Could you check a few things on this model? Use its own coordinates, in mm. A direction names the side the tool comes from. Round coordinates to 2 decimals unless told otherwise and drop trailing zeros. Loops run counter-clockwise (first coordinate to the right, second up) from the corner with the lowest first, then second, coordinate; pieces in that order, holes last. Notation, with made-up numbers: M 67,72.25 L 118,72.25 A21 ccw 118,94.25 Z; hole C -16.5,58 d10. An arc over 180 degrees is marked long. Answer in a Markdown table with one row per item.
```python
from build123d import *

# Parameters (mm, degrees)
SKETCH_1_W               = 154
SKETCH_1_H               = 37.7
EXTRUDE_1_DEPTH          = 4
CUT_EXTRUDE_1_DEPTH      = 80.374570865
CUT_EXTRUDE_1_DEPTH_BACK = 80.374570865
SKETCH_2_R               = 2
CUT_EXTRUDE_2_DEPTH      = 80.374570865
CUT_EXTRUDE_2_DEPTH_BACK = 80.374570865
FILLET_1_R               = 7
SKETCH_4_W               = 30
SKETCH_4_H               = 37.7
EXTRUDE_2_DEPTH          = 40
CUT_EXTRUDE_3_DEPTH      = 89.793707547
CUT_EXTRUDE_3_DEPTH_BACK = 89.793707547
SKETCH_5_W               = 20
SKETCH_5_H               = 11.35
CUT_EXTRUDE_4_DEPTH      = 89.793707547
CUT_EXTRUDE_4_DEPTH_BACK = 89.793707547
FILLET_2_R               = 1
FILLET_4_R               = 1


with BuildPart() as part:
    # 草图1 → 凸台-拉伸1 (new body)
    with BuildSketch(Plane(origin=(0, 0, 0), x_dir=(1, 0, 0), z_dir=(0, 1, 0))):
        Rectangle(SKETCH_1_W, SKETCH_1_H)
    extrude(amount=-EXTRUDE_1_DEPTH)

    # 草图2 → 切除-拉伸1 (cut, two sides: drawn at the far end of the back side and taken through both)
    with BuildSketch(Plane(origin=(0, 0, 0), x_dir=(1, 0, 0), z_dir=(0, 1, 0)).offset(-CUT_EXTRUDE_1_DEPTH_BACK)):
        with Locations(Location((-30, 11.85, 0), (0, 0, 270))):
            Circle(SKETCH_2_R)
        with Locations(Location((-20, -11.85, 0), (0, 0, 270))):
            Circle(SKETCH_2_R)
        with Locations(Location((-40, 11.85, 0), (0, 0, 270))):
            Circle(SKETCH_2_R)
        with Locations(Location((-50, 11.85, 0), (0, 0, 270))):
            Circle(SKETCH_2_R)
        with Locations(Location((-60, 11.85, 0), (0, 0, 270))):
            Circle(SKETCH_2_R)
        with Locations(Location((-30, -11.85, 0), (0, 0, 270))):
            Circle(SKETCH_2_R)
        with Locations(Location((-40, -11.85, 0), (0, 0, 270))):
            Circle(SKETCH_2_R)
        with Locations(Location((-50, -11.85, 0), (0, 0, 270))):
            Circle(SKETCH_2_R)
        with Locations(Location((-60, -11.85, 0), (0, 0, 270))):
            Circle(SKETCH_2_R)
        with Locations(Location((-70, -11.85, 0), (0, 0, 270))):
            Circle(SKETCH_2_R)
        with Locations(Location((20, -11.85, 0), (0, 0, 270))):
            Circle(SKETCH_2_R)
        with Locations(Location((30, -11.85, 0), (0, 0, 270))):
            Circle(SKETCH_2_R)
        with Locations(Location((40, -11.85, 0), (0, 0, 270))):
            Circle(SKETCH_2_R)
        with Locations(Location((50, -11.85, 0), (0, 0, 270))):
            Circle(SKETCH_2_R)
        with Locations(Location((60, -11.85, 0), (0, 0, 270))):
            Circle(SKETCH_2_R)
        with Locations(Location((70, -11.85, 0), (0, 0, 270))):
            Circle(SKETCH_2_R)
        with Locations(Location((30, 11.85, 0), (0, 0, 270))):
            Circle(SKETCH_2_R)
        with Locations(Location((40, 11.85, 0), (0, 0, 270))):
            Circle(SKETCH_2_R)
        with Locations(Location((50, 11.85, 0), (0, 0, 270))):
            Circle(SKETCH_2_R)
        with Locations(Location((60, 11.85, 0), (0, 0, 270))):
            Circle(SKETCH_2_R)
    extrude(amount=CUT_EXTRUDE_1_DEPTH + CUT_EXTRUDE_1_DEPTH_BACK, mode=Mode.SUBTRACT)

    # 草图3 → 切除-拉伸2 (cut, two sides: drawn at the far end of the back side and taken through both)
    with BuildSketch(Plane(origin=(0, 0, 0), x_dir=(1, 0, 0), z_dir=(0, 1, 0)).offset(-CUT_EXTRUDE_2_DEPTH_BACK)):
        Polygon((-64.644023205, 18.85), (-77, -10.433665004), (-77, 18.85), align=None)
        Polygon((64.644023205, 18.85), (77, -10.433665004), (77, 18.85), align=None)
    extrude(amount=CUT_EXTRUDE_2_DEPTH + CUT_EXTRUDE_2_DEPTH_BACK, mode=Mode.SUBTRACT)

    # 圆角1
    fillet_1_edges = [part.edges().sort_by_distance(p)[0] for p in [
        (77, -2, 18.85),
        (77, -2, 10.433665004),
        (64.644023205, -2, -18.85),
        (-77, -2, 18.85),
        (-77, -2, 10.433665004),
        (-64.644023205, -2, -18.85),
    ]]
    fillet(fillet_1_edges, radius=FILLET_1_R - 0.0001)  # a hair under: the kernel refuses the full size

    # 草图4 → 凸台-拉伸2 (add)
    with BuildSketch(Plane(origin=(0, 0, 0), x_dir=(1, 0, 0), z_dir=(0, 1, 0))):
        Rectangle(SKETCH_4_W, SKETCH_4_H)
    extrude(amount=EXTRUDE_2_DEPTH)

    # 草图5 → 切除-拉伸3 (cut, two sides: drawn at the far end of the back side and taken through both)
    with BuildSketch(Plane(origin=(0, 0, 0), x_dir=(1, 0, 0), z_dir=(0, 1, 0)).offset(-CUT_EXTRUDE_3_DEPTH_BACK)):
        with Locations((0, 8.175)):
            Rectangle(SKETCH_5_W, SKETCH_5_H)
        with Locations((0, -8.175)):
            Rectangle(SKETCH_5_W, SKETCH_5_H)
    extrude(amount=CUT_EXTRUDE_3_DEPTH + CUT_EXTRUDE_3_DEPTH_BACK, mode=Mode.SUBTRACT)

    # 草图6 → 切除-拉伸4 (cut, two sides: drawn at the far end of the back side and taken through both)
    with BuildSketch(Plane(origin=(0, 0, 0), x_dir=(1, 0, 0), z_dir=(0, 1, 0)).offset(-CUT_EXTRUDE_4_DEPTH_BACK)):
        Polygon((-34.341491259, -6.705332858), (-40, 6.705332858), (-45.658508741, -6.705332858), align=None)
        Polygon((-55.658508741, 6.705332858), (-50, -6.705332858), (-44.341491259, 6.705332858), align=None)
        Polygon((-60, 6.705332858), (-65.658508741, -6.705332858), (-54.341491259, -6.705332858), align=None)
        Polygon((-35.658508741, 6.705332858), (-30, -6.705332858), (-24.341491259, 6.705332858), align=None)
        Polygon((24.341491259, 6.705332858), (35.658508741, 6.705332858), (30, -6.705332858), align=None)
        Polygon((45.658508741, -6.705332858), (34.341491259, -6.705332858), (40, 6.705332858), align=None)
        Polygon((44.341491259, 6.705332858), (55.658508741, 6.705332858), (50, -6.705332858), align=None)
        Polygon((65.658508741, -6.705332858), (54.341491259, -6.705332858), (60, 6.705332858), align=None)
    extrude(amount=CUT_EXTRUDE_4_DEPTH + CUT_EXTRUDE_4_DEPTH_BACK, mode=Mode.SUBTRACT)

    # 圆角2
    fillet_2_edges = [part.edges().sort_by_distance(p)[0] for p in [
        (50, -2, 6.705332858),
        (44.341491259, -2, -6.705332858),
        (55.658508741, -2, -6.705332858),
        (40, -2, -6.705332858),
        (45.658508741, -2, 6.705332858),
        (34.341491259, -2, 6.705332858),
        (60, -2, -6.705332858),
        (65.658508741, -2, 6.705332858),
        (54.341491259, -2, 6.705332858),
        (-45.658508741, -2, 6.705332858),
        (-40, -2, -6.705332858),
        (-34.341491259, -2, 6.705332858),
        (-60, -2, -6.705332858),
        (-54.341491259, -2, 6.705332858),
        (-65.658508741, -2, 6.705332858),
        (-24.341491259, -2, -6.705332858),
        (-30, -2, 6.705332858),
        (-35.658508741, -2, -6.705332858),
        (-44.341491259, -2, -6.705332858),
        (-50, -2, 6.705332858),
        (-55.658508741, -2, -6.705332858),
        (30, -2, 6.705332858),
        (24.341491259, -2, -6.705332858),
        (35.658508741, -2, -6.705332858),
    ]]
    fillet(fillet_2_edges, radius=FILLET_2_R)

    # 圆角4
    fillet_4_edges = [part.edges().sort_by_distance(p)[0] for p in [
        (-15, 0, 0),
        (15, 0, 0),
    ]]
    fillet(fillet_4_edges, radius=FILLET_4_R)


solid = part.part
```
1) If we mould it in two halves opening along X, with no side actions, what happens to faces 1 (the face through (-10, 18, -8)), 2 (the face through (0, 13, 18.85)), 3 (the face through (15, 20, 0))? For each: released by +X, released by -X, zero draft, split by the parting line, or undercut.
Computed:
| item | result |
|---|---|
| face 1 | undercut |
| face 2 | zero draft |
| face 3 | released by +X |
2) I need wall thicknesses on line 1 (Z direction, x = 50, y = -1); line 2 (Z direction, x = 6, y = 11.5); line 3 (X direction, y = 34.5, z = 5). Which ranges of each line are inside material? Lowest first, please.
Computed:
| item | result |
|---|---|
| line 1 | z = -18.85 to -13.85, -9.85 to -6.71, 5.13 to 9.85, 13.85 to 18.85 |
| line 2 | z = -18.85 to -13.85, -2.5 to 2.5, 13.85 to 18.85 |
| line 3 | x = -15 to -10, 10 to 15 |
3) I want a section at C-C, the plane z = -12. State how many separate pieces and enclosed holes the cut face has, plus the area to 3 significant figures.
Computed:
| item | result |
|---|---|
| separate pieces | 10 |
| enclosed holes | 0 |
| area | 733 mm² |
4) Which directions (+Z, -Z, +X, -X, +Y, -Y) give clear straight access to the entire face, cutting with the end or side of a thin tool? Please do faces 4 (the face through (42.97, -2.03, 0.33)), 5 (the face through (-71.38, -2.03, -2.89)).
Computed:
| item | result |
|---|---|
| face 4 | +Y, -Y |
| face 5 | -Z, -X, +Y, -Y |
5) Will these pins go through, and if not, where does the flat tip stop? P1, Ø3, axis at x = -40, z = 11.85, coming from the -Y side; P2, Ø12, axis at x = -16.5, y = 15.5, coming from the -Z side; P3, Ø3.5, axis at y = 10, z = 8, coming from the -X side; P4, Ø12.5, axis at y = 9, z = 8, coming from the +X side.
Computed:
| item | result |
|---|---|
| P1 | passes through |
| P2 | stops at z = -18.85 |
| P3 | stops at x = -15 |
| P4 | stops at x = 15 |
6) I want a section at B-B, the plane y = 11. Please give me the cut outline in (x, z).
Computed:
| item | result |
|---|---|
| outline | M -15,-18.85 L 15,-18.85 L 15,18.85 L -15,18.85 Z; hole M -10,-13.85 L 10,-13.85 L 10,-2.5 L -10,-2.5 Z; hole M -10,2.5 L 10,2.5 L 10,13.85 L -10,13.85 Z |
7) I want a section at A-A, the plane x = -6. Please give me the cut outline in (y, z), plus the area to 3 significant figures.
Computed:
| item | result |
|---|---|
| outline | M -4,-18.85 L 40,-18.85 L 40,-13.85 L -4,-13.85 Z; M -4,-2.5 L 40,-2.5 L 40,2.5 L -4,2.5 Z; M -4,13.85 L 40,13.85 L 40,18.85 L -4,18.85 Z |
| area | 660 mm² |
